```python
from build123d import *

# Parameters (mm, degrees)
SKETCH1_R           = 1.5
BOSS_EXTRUDE1_DEPTH = 2
SKETCH10_W          = 16
SKETCH10_H          = 30
BOSS_EXTRUDE2_DEPTH = 29.5
FILLET1_R           = 1
SKETCH11_R          = 2.5
CUT_EXTRUDE1_DEPTH  = 32.5
BOSS_EXTRUDE4_DEPTH = 30


with BuildPart() as part:
    # Sketch1 → Boss-Extrude1 (new body)
    # profile 1 of 5: a face of its own
    with BuildSketch(Plane(origin=(0, 0, 0), x_dir=(1, 0, 0), z_dir=(0, 1, 0))):
        with BuildLine():
            Line((-15, -7), (-15, -15))
            Line((-15, -15), (-7, -15))
            ThreePointArc((-7, -15), (-9.343145751, -9.343145751), (-15, -7))
        make_face()
        with Locations(Location((-12, -12, 0), (0, 0, 270))):
            Circle(SKETCH1_R, mode=Mode.SUBTRACT)
    # profile 2 of 5: a face of its own
    with BuildSketch(Plane(origin=(0, 0, 0), x_dir=(1, 0, 0), z_dir=(0, 1, 0))):
        with BuildLine():
            ThreePointArc((15, -7), (9.343145751, -9.343145751), (7, -15))
            Line((7, -15), (15, -15))
            Line((15, -15), (15, -7))
        make_face()
        with Locations(Location((12, -12, 0), (0, 0, 270))):
            Circle(SKETCH1_R, mode=Mode.SUBTRACT)
    # profile 3 of 5: a face of its own
    with BuildSketch(Plane(origin=(0, 0, 0), x_dir=(1, 0, 0), z_dir=(0, 1, 0))):
        with BuildLine():
            ThreePointArc((-15, -7), (-9.343145751, -9.343145751), (-7, -15))
            Line((-7, -15), (7, -15))
            ThreePointArc((7, -15), (9.343145751, -9.343145751), (15, -7))
            Line((15, -7), (15, 7))
            ThreePointArc((15, 7), (9.343145751, 9.343145751), (7, 15))
            Line((7, 15), (-7, 15))
            ThreePointArc((-7, 15), (-9.343145751, 9.343145751), (-15, 7))
            Line((-15, 7), (-15, -7))
        make_face()
    # profile 4 of 5: a face of its own
    with BuildSketch(Plane(origin=(0, 0, 0), x_dir=(1, 0, 0), z_dir=(0, 1, 0))):
        with BuildLine():
            ThreePointArc((7, 15), (9.343145751, 9.343145751), (15, 7))
            Line((15, 7), (15, 15))
            Line((15, 15), (7, 15))
        make_face()
        with Locations(Location((12, 12, 0), (0, 0, 270))):
            Circle(SKETCH1_R, mode=Mode.SUBTRACT)
    # profile 5 of 5: a face of its own
    with BuildSketch(Plane(origin=(0, 0, 0), x_dir=(1, 0, 0), z_dir=(0, 1, 0))):
        with BuildLine():
            Line((-15, 15), (-15, 7))
            ThreePointArc((-15, 7), (-9.343145751, 9.343145751), (-7, 15))
            Line((-7, 15), (-15, 15))
        make_face()
        with Locations(Location((-12, 12, 0), (0, 0, 270))):
            Circle(SKETCH1_R, mode=Mode.SUBTRACT)
    extrude(amount=BOSS_EXTRUDE1_DEPTH)

    # Sketch10 → Boss-Extrude2 (add)
    with BuildSketch(Plane(origin=(0, 2, 0), x_dir=(1, 0, 0), z_dir=(0, 1, 0))):
        Rectangle(SKETCH10_W, SKETCH10_H)
    extrude(amount=BOSS_EXTRUDE2_DEPTH)

    # Fillet1
    fillet1_edges = [part.edges().sort_by_distance(p)[0] for p in [
        (-8, 2, 0),
        (8, 2, 0),
    ]]
    fillet(fillet1_edges, radius=FILLET1_R)

    # Sketch11 → Cut-Extrude1 (cut)
    with BuildSketch(Plane.XY.offset(15)):
        with Locations((0, 21.5)):
            Circle(SKETCH11_R)
    extrude(amount=-CUT_EXTRUDE1_DEPTH, mode=Mode.SUBTRACT)

    # Sketch13 → Boss-Extrude4 (add)
    with BuildSketch(Plane.XY.offset(15)):
        Polygon((-4.75, 34.2), (-3, 34.2), (-3, 33.3), (-3, 33.25), (-3, 31.5), (3, 31.5), (3, 33.25), (3, 33.3), (3, 34.2), (4.75, 34.2), (4.75, 35.689339828), (3.139339828, 37.3), (0.1, 37.3), (0, 37.4), (-0.1, 37.3), (-3.139339828, 37.3), (-4.75, 35.689339828), align=None)
    extrude(amount=-BOSS_EXTRUDE4_DEPTH)


solid = part.part
```
Work out the finished part from the listing and answer in its coordinate system (mm). A direction names the side the tool comes from. Coordinates: 2 decimals unless noted, no trailing zeros. Order: outer loops, then holes, each group sorted by start corner. A loop starts at its lowest first (then second) coordinate and runs counter-clockwise, first axis right, second up. Notation, with made-up numbers: M 9.5,73 L 43.5,73 A11 cw 43.5,92 Z; hole C -21,55.25 d9. An arc over 180 degrees is marked long. Use CSV: the item, a comma, the result in double quotes.
1) Section D-D on z = 1 is taken. Write down the section's boundary in (x, y).
Worked out:
outline,"M -15,0 L 15,0 L 15,2 L 9,2 A1 cw 8,3 L 8,31.5 L 3,31.5 L 3,34.2 L 4.75,34.2 L 4.75,35.69 L 3.14,37.3 L 0.1,37.3 L 0,37.4 L -0.1,37.3 L -3.14,37.3 L -4.75,35.69 L -4.75,34.2 L -3,34.2 L -3,31.5 L -8,31.5 L -8,3 A1 cw -9,2 L -15,2 Z; hole C 0,21.5 d5"
2) Section B-B on z = 12 is taken. Count the separate pieces of the cut face and the enclosed holes in it, plus the area to 3 significant figures.
Worked out:
separate pieces,"3"
enclosed holes,"1"
area,"544 mm^2"
3) For faces 1 (the face through (-6, 31.5, 0)), 2 (the face through (8, 17, 0)), 3 (the face through (-2, 37.3, 0)), determine the directions among +Z, -Z, +X, -X, +Y, -Y from which every point of the face is accessible in a straight line to the end or side of a thin tool.
Worked out:
face 1,"+Z, -Z, -X"
face 2,"+Z, -Z, +X, +Y"
face 3,"+Z, -Z, -X, +Y"
4) Section A-A on x = 12 is taken. Write down the section's boundary in (y, z), plus the area to 3 significant figures.
Worked out:
outline,"M 0,-15 L 2,-15 L 2,-13.5 L 0,-13.5 Z; M 0,-10.5 L 2,-10.5 L 2,10.5 L 0,10.5 Z; M 0,13.5 L 2,13.5 L 2,15 L 0,15 Z"
area,"48.0 mm^2"
5) Consider line 1 (X direction, y = 0.5, z = 12); line 2 (X direction, y = 5, z = 2); line 3 (Y direction, x = -3.25, z = -9.75). Determine where each line is inside the solid, lowest interval first. Write a range as [from, to].
Worked out:
line 1,"x = [-15, -13.5], [-10.5, 10.5], [13.5, 15]"
line 2,"x = [-8, 8]"
line 3,"y = [0, 31.5], [34.2, 37.19]"
6) Determine the mould class of faces 4 (the face through (5, 31.5, 0)), 5 (the face through (8.301, 2.285, -0.21)), 6 (the face through (3, 33, 0)), 7 (the face through (15, 1, 0)) for opening direction Y: released by +Y, released by -Y, zero draft, split by the parting line, or undercut.
Worked out:
face 4,"undercut"
face 5,"released by +Y"
face 6,"undercut"
face 7,"zero draft"
7) Flat-ended cylindrical pins translate along their axes: pin 1 Ø14 at (y, z) = (11.5, -3) entering from +X; pin 2 Ø1.6 at (y, z) = (35, -1) entering from -X; pin 3 Ø8 at (y, z) = (19.5, -7) entering from -X. Find the tip coordinate at first contact, or state that the pin passes through.
Worked out:
pin 1,"stops at x = 8"
pin 2,"stops at x = -4.75"
pin 3,"stops at x = -8"
8) Section C-C on y = 21.5 is taken. Write down the section's boundary in (x, z).
Worked out:
outline,"M -8,-15 L -2.5,-15 L -2.5,15 L -8,15 Z; M 2.5,-15 L 8,-15 L 8,15 L 2.5,15 Z"
